CAD build for the part. Positions are in the model's coordinates, mm. Face numbers are marked on the shaded views. A direction names the side the tool comes from. Give positions to 0.01 mm unless a question says otherwise; leave off trailing zeros. Loops run counter-clockwise (first coordinate to the right, second up) from the corner with the lowest first, then second, coordinate; pieces in that order, holes last. Notation, with made-up numbers: (-25.75, 70.5) - (23.25, 70.5) arc R14 cw to (23.25, 84.5) - close; hole circle Ø5 at (-25.5, 85). An arc over 180 degrees is marked (long way). Return JSON: item names as keys, results as strings.
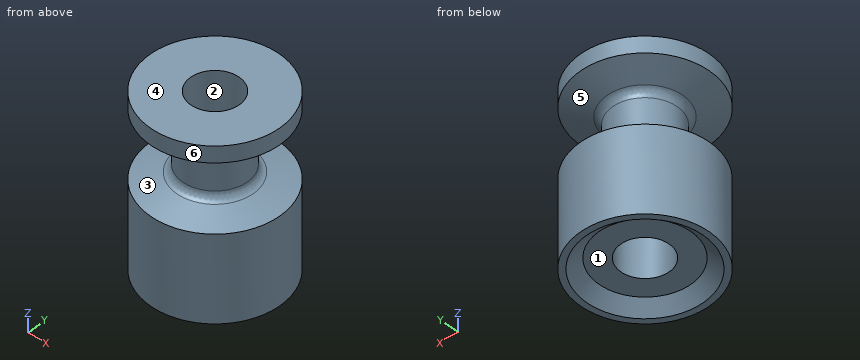
from build123d import *

# Parameters (mm, degrees)
SKETCH_1_R      = 4
SKETCH_1_R_2    = 1.5
EXTRUDE_1_DEPTH = 10.5
FILLET_1_R      = 0.5


with BuildPart() as part:
    # 草图1 → 凸台-拉伸1 (new body)
    with BuildSketch(Plane.XY):
        with Locations(Location((0, 0, 0), (0, 0, 180))):
            Circle(SKETCH_1_R)
        with Locations(Location((0, 0, 0), (0, 0, 180))):
            Circle(SKETCH_1_R_2, mode=Mode.SUBTRACT)
    extrude(amount=EXTRUDE_1_DEPTH)

    # 草图3 → 切除-旋转1 (revolve, cut)
    with BuildSketch(Plane(origin=(0, 0, 0), x_dir=(1, 0, 0), z_dir=(0, 1, 0))):
        Polygon((-3.624639835, 0), (-2.85, -0.65), (0, -0.65), (0, 0), align=None)
        Polygon((-4, -5.3), (-4, -9.5), (-2, -8.850160608), (-2, -5.835898385), align=None)
    revolve(axis=Axis((0, 0, 0), (0, 0, 1)), mode=Mode.SUBTRACT)

    # 圆角1
    fillet_1_edges = [part.edges().sort_by_distance(p)[0] for p in [
        (2, 0, 5.835898385),
        (2, 0, 8.850160608),
    ]]
    fillet(fillet_1_edges, radius=FILLET_1_R)


solid = part.part
1. Cut at B-B, the plane z = 7.5. Write the cut outline in (x, y), plus the area to 3 significant figures.
Values follow:
{"outline": "circle Ø4 at (0, 0); hole circle Ø3 at (0, 0)", "area": "5.50 mm²"}
2. Drill centre lines: probe 1 along Y at (x, z) = (0, 7); probe 2 along Y at (x, z) = (0, 3.5); probe 3 along Z at (x, y) = (2, 0.75). Where is each one in solid material? Low to high.
Values follow:
{"probe 1": "y = -2 to -1.5, 1.5 to 2", "probe 2": "y = -4 to -1.5, 1.5 to 4", "probe 3": "z = 0.65 to 5.88, 8.83 to 10.5"}
3. Which spindle directions (+Z, -Z, +X, -X, +Y, -Y) get a long thin tool onto all of the face, cutting with end or side? Do the marked faces 1, 2 and 3. Say none if no direction does.
Values follow:
{"face 1": "-Z", "face 2": "+Z, -Z", "face 3": "none"}
4. Pull direction Z, two halves, no side cores. Call the marked faces 4, 5 and 6: +Z half, -Z half, draft (parallel to the pull), parting line (faces both ways), or undercut.
Values follow:
{"face 4": "+Z half", "face 5": "undercut", "face 6": "draft"}
5. Drop flat-ended pins along their axis: P1, Ø1.5, axis at y = -1.5, z = 8, coming from the -X side; P2, Ø2, axis at y = 0.5, z = 3, coming from the -X side. Give the stop position or say it passes through.
Values follow:
{"P1": "stops at x = -1.85", "P2": "stops at x = -4"}
6. Cut at A-A, the plane z = 4. Write the cut outline in (x, y).
Values follow:
{"outline": "circle Ø8 at (0, 0); hole circle Ø3 at (0, 0)"}
